from build123d import *

# Parameters (mm, degrees)
F0_W     = 120
F0_H     = 30
F1_DEPTH = 5
F3_DEPTH = 1390
F4_W     = 120
F4_H     = 30
F5_DEPTH = 5
F6_R     = 4
F7_DEPTH = 25
F8_R     = 4
F9_DEPTH = 25


with BuildPart() as f1:
    # F0 (on Top) → F1 (new body)
    with BuildSketch(Plane.XY):
        Rectangle(F0_W, F0_H)
    extrude(amount=F1_DEPTH)

    # F2 (on face) → F3 (join)
    with BuildSketch(Plane.XY.offset(5)):
        Polygon((-55, 15), (-60, 15), (-60, -15), (-30, -15), (-30, -10), (-55, -10), align=None)
    extrude(amount=F3_DEPTH)

    # F4 (on face) → F5 (join)
    with BuildSketch(Plane.XY.offset(1395)):
        Rectangle(F4_W, F4_H)
    extrude(amount=F5_DEPTH)

    # F6 (on face) → F7 (cut)
    with BuildSketch(Plane.XY.offset(1400)):
        with Locations((36.882059, 0)):
            Circle(F6_R)
    extrude(amount=-F7_DEPTH, mode=Mode.SUBTRACT)

    # F8 (on face) → F9 (cut)
    with BuildSketch(Plane.XY.offset(5)):
        with Locations((34.570879, 0)):
            Circle(F8_R)
    extrude(amount=-F9_DEPTH, mode=Mode.SUBTRACT)


solid = f1.part
The listing builds one solid part. Answer for the finished solid, in the listing's coordinates (mm). A direction names the side the tool comes from. Round coordinates to 2 decimals unless told otherwise and drop trailing zeros. Order: outer loops, then holes, each group sorted by start corner. A loop starts at its lowest first (then second) coordinate and runs counter-clockwise, first axis right, second up. Notation, with made-up numbers: (45.5, 10) -> (66.5, 10) arc R23 cw to (66.5, 29) -> close; hole circle Ø5 at (-1, 69). An arc over 180 degrees is marked (long way). One line per item, written item: value.
Item 1: Given P1, Ø7.5, axis at y = -1, z = 802, coming from the +X side; P2, Ø2.5, axis at y = -12.5, z = 772, coming from the +X side; P3, Ø5, axis at x = 36.88, y = 0, coming from the +Z side, each flat-ended and moving along its own axis, determine where each tip first touches the part or whether it passes through.
Taken from the geometry:
P1: stops at x = -55
P2: stops at x = -30
P3: stops at z = 5
Item 2: For faces 1 (the flat face through (-60, 0, 690)), 2 (the flat face through (2, 0, 1395)), determine the directions among +Z, -Z, +X, -X, +Y, -Y from which every point of the face is accessible in a straight line to the end or side of a thin tool.
Taken from the geometry:
face 1: +Z, -Z, -X, +Y, -Y
face 2: +X, +Y
Item 3: Find section B-B, the plane z = 1230.5. Give the vertices of the cut face in (x, y), then the cut area to 3 significant figures.
Taken from the geometry:
outline: (-60, -15) -> (-30, -15) -> (-30, -10) -> (-55, -10) -> (-55, 15) -> (-60, 15) -> close
area: 275 mm2
Item 4: Find section A-A, the plane x = 17. Give the vertices of the cut face in (y, z), then the cut area to 3 significant figures.
Taken from the geometry:
outline: (-15, 0) -> (15, 0) -> (15, 5) -> (-15, 5) -> close; (-15, 1395) -> (15, 1395) -> (15, 1400) -> (-15, 1400) -> close
area: 300 mm2
Item 5: Straight lines are drawn through the part: L1, parallel to Z at x = 32, y = 4.5; L2, parallel to X at y = -9.75, z = 1005; L3, parallel to Z at x = 37, y = 3.75. For each, find the intervals that lie inside material, in ascending order.
Taken from the geometry:
L1: z = 0 to 5, 1395 to 1400
L2: x = -60 to -55
L3: z = 0 to 5
Item 6: For a pull along Z with two mould halves and no side action, classify faces 3 (the flat face through (-1, 0, 1400)), 4 (the flat face through (-58, 15, 697)), 5 (the flat face through (2, 0, 5)), 6 (the flat face through (-55, 2, 690)) as released by +Z, released by -Z, zero draft, split by the parting line, or undercut.
Taken from the geometry:
face 3: released by +Z
face 4: zero draft
face 5: undercut
face 6: undercut
